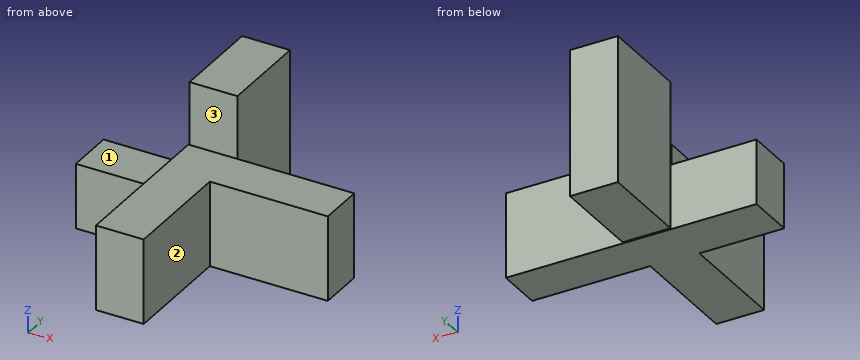
from build123d import *

# Parameters (mm, degrees)
F0_W     = 14.2970732413
F0_H     = 34.1241974384
F0_H_2   = 13.6066358536
F0_W_2   = 35.348333884
F1_DEPTH = 12.7
F2_W     = 14.3289165571
F2_H     = 43.9045364037
F3_DEPTH = 27.178
F4_W     = 14.3301561475
F4_H     = 19.4006666213
F5_DEPTH = 25.4


with BuildPart() as f1:
    # F0 (on Top) → F1 (new body, symmetric)
    with BuildSketch(Plane.XY):
        with Locations((-13.6043701787, -30.6687345728)):
            Rectangle(F0_W, F0_H)
        with Locations((-13.6043701787, -6.8033179268)):
            Rectangle(F0_W, F0_H_2)
        with Locations((11.218333384, -6.8033179268)):
            Rectangle(F0_W_2, F0_H_2)
    extrude(amount=F1_DEPTH, both=True)

    # F2 (on Front) → F3 (join)
    with BuildSketch(Plane.XZ):
        with Locations((-13.2477167062, 9.6126752906)):
            Rectangle(F2_W, F2_H)
    extrude(amount=-F3_DEPTH)

    # F4 (on face) → F5 (join)
    with BuildSketch(Plane(origin=(-20.7529067993, 0, 0), x_dir=(0, -1, 0), z_dir=(-1, 0, 0))):
        with Locations((7.1650780737, -2.9996666893)):
            Rectangle(F4_W, F4_H)
    extrude(amount=F5_DEPTH)


solid = f1.part
Work out the finished part from the listing and answer in its coordinate system (mm). Face numbers are marked on the shaded views. A direction names the side the tool comes from. Coordinates: 2 decimals unless noted, no trailing zeros. Write each loop counter-clockwise with the first axis right and the second up, starting at its lowest first coordinate (ties: lowest second). Pieces come first, ordered by that corner, then holes. Notation, with made-up numbers: M -25,-18.75 L 23,-18.75 A19 ccw 23,-6.75 Z; hole C 62,-19 d2. An arc over 180 degrees is marked long. Use one line per item in the form item = value. Start each with the question number.
1. The part is cut by section C-C (x = -9.5). Give the vertices of the cut face in (y, z).
2. The part is cut by section D-D (y = -22). Give the vertices of the cut face in (x, z).
3. A tool of negligible diameter and unlimited length cuts with its end or side. For the marked faces 1, 2 and 3, from which of +Z, -Z, +X, -X, +Y, -Y can it reach the whole face along a straight path? Write none if from no direction.
4. Each of these flat-tipped pins is pushed along its axis until it touches: P1, Ø4, axis at y = -29.5, z = 3.5, coming from the +X side; P2, Ø5, axis at x = -18, y = -24, coming from the +Z side; P3, Ø3, axis at y = -9, z = 11.5, coming from the -X side; P4, Ø3, axis at x = -3.5, z = 23.5, coming from the +Y side. Where does it stop, or does it pass through?
5. The part is cut by section B-B (y = -4). Give the vertices of the cut face in (x, z).
6. Straight lines are drawn through the part: probe 1 along X at (y, z) = (-17, -7); probe 2 along Y at (x, z) = (-2, 3.5); probe 3 along Y at (x, z) = (-28, -7.5). For each, find the intervals that lie inside material, in ascending order. Write a range as from..to.
7. The part is cut by section A-A (z = -2). Give the vertices of the cut face in (x, y), plus the area to 3 significant figures.
Evaluation:
q1.outline = M -47.73,-12.7 L 0,-12.7 L 0,-12.34 L 27.18,-12.34 L 27.18,31.56 L 0,31.56 L 0,12.7 L -47.73,12.7 Z
q2.outline = M -20.75,-12.7 L -6.46,-12.7 L -6.46,12.7 L -20.75,12.7 Z
q3.face_1 = +Z, -X, +Y, -Y
q3.face_2 = +Z, -Z, +X, -Y
q3.face_3 = +Z, +X, -X, -Y
q4.P1 = -6.46
q4.P2 = 12.7
q4.P3 = -20.75
q4.P4 = through
q5.outline = M -46.15,-12.7 L 28.89,-12.7 L 28.89,12.7 L -20.75,12.7 L -20.75,6.7 L -46.15,6.7 Z
q6.probe_1 = -20.75..-6.46
q6.probe_2 = -13.61..0
q6.probe_3 = -14.33..0
q7.outline = M -46.15,-14.33 L -20.75,-14.33 L -20.75,-47.73 L -6.46,-47.73 L -6.46,-13.61 L 28.89,-13.61 L 28.89,0 L -6.08,0 L -6.08,27.18 L -20.41,27.18 L -20.41,0 L -46.15,0 Z
q7.area = 1,920 mm^2
